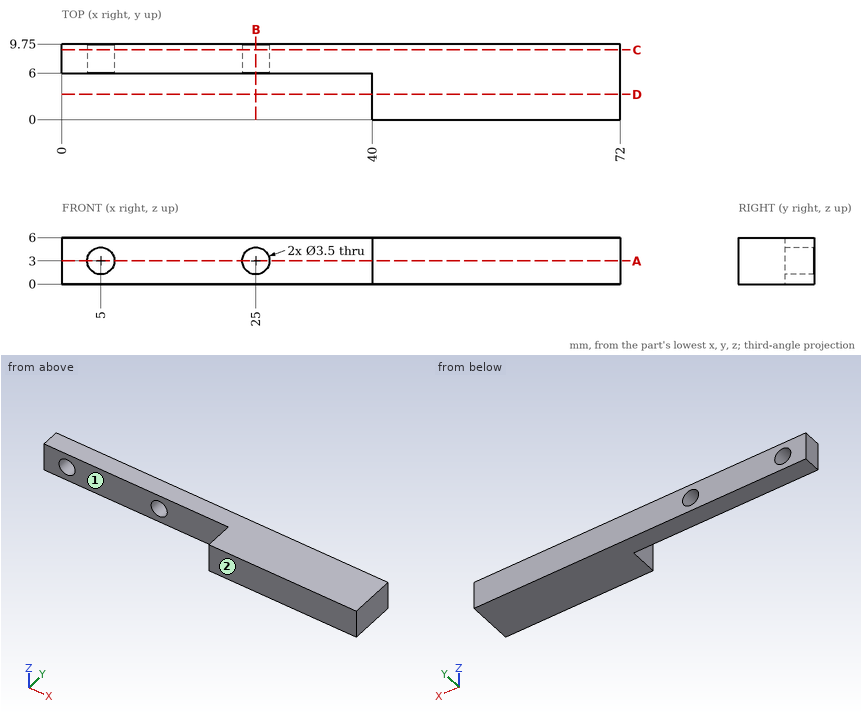
The drawing under review shows one solid part. Ordinate dimensions are in mm from its lowest x, y, z. A direction names the side the tool comes from. Give positions to 0.01 mm unless a question says otherwise; leave off trailing zeros. Write each loop counter-clockwise with the first axis right and the second up, starting at its lowest first coordinate (ties: lowest second). Pieces come first, ordered by that corner, then holes. Notation, with made-up numbers: (-40, 70.25) - (-7, 70.25) arc R4 cw to (-7, 75.25) - close; hole circle Ø6 at (41, 45). An arc over 180 degrees is marked (long way). Answer in a Markdown table with one row per item. Add a question column.
1. We need section A-A on z = 3. Write out the cut boundary in (x, y), then the cut area to 3 significant figures.
2. We need section D-D on y = 3.25. Write out the cut boundary in (x, z), then the cut area to 3 significant figures.
3. Tool access review of the marked faces 1 and 2: name each direction out of +Z, -Z, +X, -X, +Y, -Y from which nothing blocks a thin tool from reaching the whole face with its end or side.
4. Wall thickness on line 1 along X through (y, z) = (8.55, 3); line 2 along X through (y, z) = (7.75, 3.85); line 3 along Y through (x, z) = (12.5, 2.1): over which ranges is each line inside the solid? List them lowest first. Write a range as [from, to].
5. We need section C-C on y = 9. Write out the cut boundary in (x, z).
6. Insertion check: P1, Ø2, axis at x = 21, z = 4, coming from the -Y side; P2, Ø1.8, axis at y = 2.5, z = 3, coming from the -X side. Each pin has a flat end and moves straight along its axis. Give the tip position at first contact, or say it passes through.
7. We need section B-B on x = 25. Write out the cut boundary in (y, z), then the cut area to 4 significant figures.
Ans:
| question | item | result |
|---|---|---|
| 1 | outline | (0, 6) - (3.25, 6) - (3.25, 9.75) - (0, 9.75) - close; (6.75, 6) - (23.25, 6) - (23.25, 9.75) - (6.75, 9.75) - close; (26.75, 6) - (40, 6) - (40, 0) - (72, 0) - (72, 9.75) - (26.75, 9.75) - close |
| 1 | area | 436 mm^2 |
| 2 | outline | (40, 0) - (72, 0) - (72, 6) - (40, 6) - close |
| 2 | area | 192 mm^2 |
| 3 | face 1 | +Z, -Z, -X, -Y |
| 3 | face 2 | +Z, -Z, +X, -X, -Y |
| 4 | line 1 | x = [0, 3.25], [6.75, 23.25], [26.75, 72] |
| 4 | line 2 | x = [0, 3.47], [6.53, 23.47], [26.53, 72] |
| 4 | line 3 | y = [6, 9.75] |
| 5 | outline | (0, 0) - (72, 0) - (72, 6) - (0, 6) - close; hole circle Ø3.5 at (5, 3); hole circle Ø3.5 at (25, 3) |
| 6 | P1 | stops at y = 6 |
| 6 | P2 | stops at x = 40 |
| 7 | outline | (6, 0) - (9.75, 0) - (9.75, 1.25) - (6, 1.25) - close; (6, 4.75) - (9.75, 4.75) - (9.75, 6) - (6, 6) - close |
| 7 | area | 9.375 mm^2 |
